Check sheet for the modelled part. Datum: model origin and axes. Units: mm. Face numbers are marked on the shaded views. A direction names the side the tool comes from. Give positions to 0.01 mm unless a question says otherwise; leave off trailing zeros. Write each loop counter-clockwise with the first axis right and the second up, starting at its lowest first coordinate (ties: lowest second). Pieces come first, ordered by that corner, then holes. Notation, with made-up numbers: M 21.5,43 L 32.5,43 A14 cw 32.5,58 Z; hole C -40,87.5 d11. An arc over 180 degrees is marked long. Write item = value, one per line. Start each with the question number.
1) Sectioned sample at C-C, the plane y = -3.75. Record the cut outline in (x, z).
2) Sectioned sample at B-B, the plane z = -73.5. Record the cut outline in (x, y).
3) Set-up check for the marked faces 1 and 2: record each of +Z, -Z, +X, -X, +Y, -Y from which the full face is reachable in a straight line by a thin tool's end or side.
4) Scan lines: L1, parallel to Z at x = -0.75, y = -3; L2, parallel to Y at x = -2, z = -7.5; L3, parallel to X at y = -0.75, z = -45. Record each from-to range of solid material in increasing order.
5) Gauge pin test, flat ends, axial feed: pin 1 (4 mm diameter, centred on y = -3.5, z = -43.5, fed in from -X); pin 2 (3 mm diameter, centred on x = -4, y = 0, fed in from -Z); pin 3 (1 mm diameter, centred on x = 4, z = -13.5, fed in from +Y). Record the tip position at first contact, or that the pin passes through.
Solid Edge part; units mm, degrees
sketch "Sketch1" plane through (0, 0, 0) normal (0, 0, 1) x (1, 0, 0)
  circle A0 centre (0, 0) radius 5.8
extrude "Protrusion1" add sketch "Sketch1" along normal blind 4.15
sketch "Sketch2" plane through (0, 0, 0) normal (0, 0, -1) x (1, 0, 0)
  circle A0 centre (0, 0) radius 3
extrude "Protrusion2" add sketch "Sketch2" along normal blind 80
sketch "Sketch3" plane through (0, 0, -80) normal (0, 0, -1) x (1, 0, 0)
  circle A0 centre (0, 0) radius 2.9997
extrude "Cutout1" cut sketch "Sketch3" against normal blind 18 flip side to cut
chamfer "Chamfer_1" distance 0.45 angle 45 1 edges at (-2.9997, 0, -80)
sketch "Sketch4" plane through (0, 0, 4.15) normal (0, 0, 1) x (1, 0, 0)
  line L0 (-2.9394, 5) -> (2.9394, 5)
extrude "Cutout2" cut sketch "Sketch4" against normal up to next material side at (0, 5.05, 4.15)
pattern_circular "Pattern1" count 6 over 360 about axis through (0, 0, 4.15) along (0, 0, 1) of "Cutout2"
properties part number "118059"
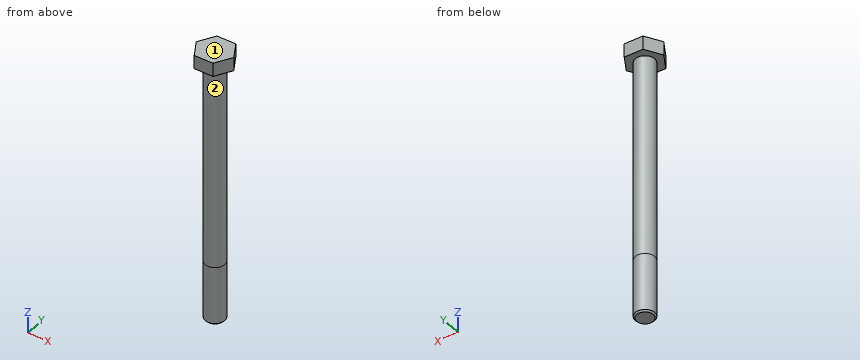
Data:
q1.outline = M -3.61,0 L 3.61,0 L 3.61,4.15 L -3.61,4.15 Z
q2.outline = C 0,0 d6
q3.face_1 = +Z, +X, -X, +Y, -Y
q3.face_2 = -Z
q4.L1 = 0 to 4.15
q4.L2 = -2.24 to 2.24
q4.L3 = -2.9 to 2.9
q5.pin_1 = -2.6
q5.pin_2 = -80
q5.pin_3 = through
